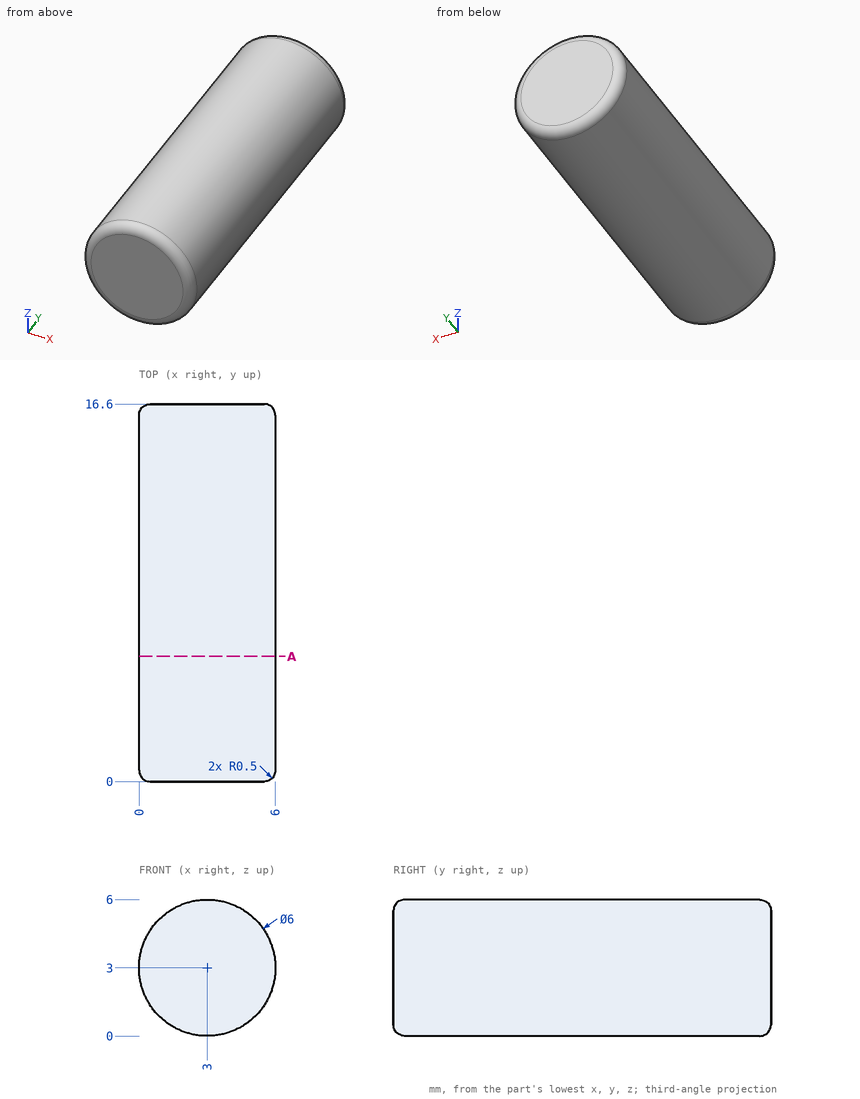
Geometry: see drawing. Coordinates: mm, zero at the bounding-box minimum. Coordinates: 2 decimals unless noted, no trailing zeros. Loops run counter-clockwise (first coordinate to the right, second up) from the corner with the lowest first, then second, coordinate; pieces in that order, holes last. Notation, with made-up numbers: (28.25, 17) -> (55.25, 17) arc R15 cw to (55.25, 28) -> close; hole circle Ø8 at (-23, -24). An arc over 180 degrees is marked (long way). Write item = value, one per line. Start each with the question number.
Item 1: Cut plane A-A, the plane y = 5.5. Return loops of the section in (x, z), plus the area to 3 significant figures.
Item 2: Material intervals for line 1 (X direction, y = 1, z = 3.1); line 2 (Y direction, x = 4.9, z = 4.7), sorted ascending.
Item 3: First-contact query: P1, Ø1, axis at x = 1, z = 1, coming from the -Y side; P2, Ø1.5, axis at x = 5, y = 6.5, coming from the -Z side. Flat tips, straight axial feed; report the tip coordinate or a pass-through.
Ans:
q1.outline = circle Ø6 at (3, 3)
q1.area = 28.3 mm²
q2.line_1 = 0 to 6
q2.line_2 = 0 to 16.6
q3.P1 = 0
q3.P2 = 0.27
